Could you check a few things on this model? Use its own coordinates, in mm. A direction names the side the tool comes from. Give positions to 0.01 mm unless a question says otherwise; leave off trailing zeros. Loops run counter-clockwise (first coordinate to the right, second up) from the corner with the lowest first, then second, coordinate; pieces in that order, holes last. Notation, with made-up numbers: (-21, -40) -> (26, -40) arc R17 ccw to (26, -20) -> close; hole circle Ø11 at (88, 53.25). An arc over 180 degrees is marked (long way). Write each question's results on one line, items separated by ' | '. Start each with the question number.
Q1. Which directions (+Z, -Z, +X, -X, +Y, -Y) give clear straight access to the entire face, cutting with the end or side of a thin tool? Please do faces 1 (the face through (0, 10, 10)), 2 (the face through (101, 45, 20)), 3 (the face through (50, 38, 10)).
Q2. We'd pull the mould along Y, two halves only. Please class faces 4 (the face through (70.85, 41.52, 9.86)), 5 (the face through (115.01, 9.86, 42.9)), 6 (the face through (76, 20, 33)): released by +Y, released by -Y, zero draft, split by the parting line, or undercut.
Q3. Will these pins go through, and if not, where does the flat tip stop? P1, Ø10, axis at y = 37.5, z = 5.5, coming from the -X side; P2, Ø11, axis at x = 75, y = 49.5, coming from the -Z side; P3, Ø1.5, axis at x = 99, y = 60.5, coming from the +Z side; P4, Ø2, axis at x = 80.5, z = 51, coming from the +Y side.
Q4. If we section it at A-A, the plane x = 75: List the corners of the cut face in (y, z) for me, plus the area to 3 significant figures.
Q5. If we section it at C-C, the plane y = 8.5: List the corners of the cut face in (x, z) for me.
Q6. If we section it at B-B, the plane z = 5: List the corners of the cut face in (x, y) for me, plus the area to 3 significant figures.
Q7. If I drill on line 1 along Z through (x, y) = (125, 12.25); line 2 along X through (y, z) = (50, 15.5); line 3 along Y through (x, z) = (75, 11.75), over which ranges is the centre line in solid material (lowest first)?
Q8. If we section it at D-D, the plane z = 34: List the corners of the cut face in (x, y) for me.
from build123d import *

# Parameters (mm, degrees)
EXTRUDE1_DEPTH            = 20
EXTRUDE2_DEPTH            = 20
FILLET1_R                 = 25
FILLET2_R                 = 20
FILLET3_R                 = 12
FILLET4_R                 = 6
M20_0_20_DIAMETER_HOLE1_D = 20
M18_0_18_DIAMETER_HOLE1_D = 18


with BuildPart() as part:
    # Sketch1 → Extrude1 (new body)
    with BuildSketch(Plane(origin=(0, 0, 0), x_dir=(1, 0, 0), z_dir=(0, 1, 0))):
        Polygon((0, 0), (150, 0), (150, -75), (0, -35), align=None)
    extrude(amount=EXTRUDE1_DEPTH)

    # Sketch2 → Extrude2 (add)
    with BuildSketch(Plane(origin=(0, 0, 0), x_dir=(-1, 0, 0), z_dir=(0, 0, -1))):
        Polygon((-150, 0), (-50, 0), (-50, 80), (-150, 60), align=None)
    extrude(amount=-EXTRUDE2_DEPTH)

    # Fillet1
    fillet1_edges = [part.edges().sort_by_distance(p)[0] for p in [
        (50, 80, 10),
        (150, 10, 75),
    ]]
    fillet(fillet1_edges, radius=FILLET1_R)

    # Fillet2
    fillet2_edges = [part.edges().sort_by_distance(p)[0] for p in [
        (0, 10, 35),
    ]]
    fillet(fillet2_edges, radius=FILLET2_R)

    # Fillet3
    fillet3_edges = [part.edges().sort_by_distance(p)[0] for p in [
        (150, 60, 10),
    ]]
    fillet(fillet3_edges, radius=FILLET3_R)

    # Fillet4
    fillet4_edges = [part.edges().sort_by_distance(p)[0] for p in [
        (50, 20, 10),
        (100, 20, 20),
    ]]
    fillet(fillet4_edges, radius=FILLET4_R)

    # M20.0 (20) Diameter Hole1 (through all)
    with Locations(Plane(origin=(0, 20, 0), x_dir=(-1, 0, 0), z_dir=(0, 1, 0))):
        with Locations((-125, 42.45970884), (-20, 19.634433738)):
            Hole(M20_0_20_DIAMETER_HOLE1_D / 2)

    # M18.0 (18) Diameter Hole1 (through all)
    with Locations(Plane(origin=(130.879919851, 20.264222767, 20), x_dir=(1, 0, 0), z_dir=(0, 0, 1))):
        with Locations((-55.879919851, 29.240679665)):
            Hole(M18_0_18_DIAMETER_HOLE1_D / 2)


solid = part.part
Final values:
1) face 1: +Z, -Z, -X, +Y, -Y | face 2: +Z, +X, -X, +Y | face 3: +Z, -Z, -X, +Y
2) face 4: undercut | face 5: zero draft | face 6: released by +Y
3) P1: stops at x = 50 | P2: passes through | P3: stops at z = 20 | P4: stops at y = 20
4) outline: (0, 0) -> (40.5, 0) -> (40.5, 20) -> (26, 20) arc R6 cw to (20, 26) -> (20, 55) -> (0, 55) -> close; (58.5, 0) -> (74.5, 0) -> (74.5, 20) -> (58.5, 20) -> close | area: 1,840 mm²
5) outline: (0, 0) -> (150, 0) -> (150, 42.46) arc R25 ccw to (118.56, 66.62) -> (14.85, 38.96) arc R20 ccw to (0, 19.63) -> close; hole circle Ø20 at (20, 19.63); hole circle Ø20 at (125, 42.46)
6) outline: (0, 0) -> (150, 0) -> (150, 50.16) arc R12 ccw to (140.35, 61.93) -> (79.9, 74.02) arc R25 ccw to (50, 49.5) -> (50, 26) arc R6 cw to (44, 20) -> (0, 20) -> close; hole circle Ø18 at (75, 49.5) | area: 7,520 mm²
7) line 1: z = 0 to 32.46, 52.46 to 67.46 | line 2: x = 50 to 66.01, 83.99 to 150 | line 3: y = 0 to 40.5, 58.5 to 74.5
8) outline: (6.08, 0) -> (119.67, 0) -> (119.67, 20) -> (6.08, 20) -> close; (130.33, 0) -> (150, 0) -> (150, 20) -> (130.33, 20) -> close
